The listing builds one solid part. Answer for the finished solid, in the listing's coordinates (mm). Face numbers are marked on the shaded views. A direction names the side the tool comes from. Round coordinates to 2 decimals unless told otherwise and drop trailing zeros. Order: outer loops, then holes, each group sorted by start corner. A loop starts at its lowest first (then second) coordinate and runs counter-clockwise, first axis right, second up. Notation, with made-up numbers: (33, 43) - (47, 43) arc R19 ccw to (47, 73) - close; hole circle Ø10 at (-27.75, -23). An arc over 180 degrees is marked (long way). One line per item, written item: value. Start each with the question number.
1. For a pull along X with two mould halves and no side action, classify the marked faces 1, 2 and 3 as released by +X, released by -X, zero draft, split by the parting line, or undercut.
2. Section A-A, the plane x = 0 is taken. Give the vertices of the cut face in (y, z), then the cut area to 3 significant figures.
3. A tool of negligible diameter and unlimited length cuts with its end or side. For the marked faces 4 and 5, from which of +Z, -Z, +X, -X, +Y, -Y can it reach the whole face along a straight path? Write none if from no direction.
4. Flat-ended cylindrical pins translate along their axes: P1, Ø5, axis at x = 1.5, y = 9.5, coming from the -Z side; P2, Ø2, axis at y = 11.5, z = 0.5, coming from the -X side; P3, Ø1.5, axis at x = 2.5, y = 6.5, coming from the -Z side. Find the tip coordinate at first contact, or state that the pin passes through.
5. Straight lines are drawn through the part: line 1 (Y direction, x = -1, z = 3.5); line 2 (Y direction, x = 1.5, z = 0.25); line 3 (X direction, y = 15.5, z = -2). For each, find the intervals that lie inside material, in ascending order.
6. Section B-B, the plane y = 7.5 is taken. Give the vertices of the cut face in (x, z).
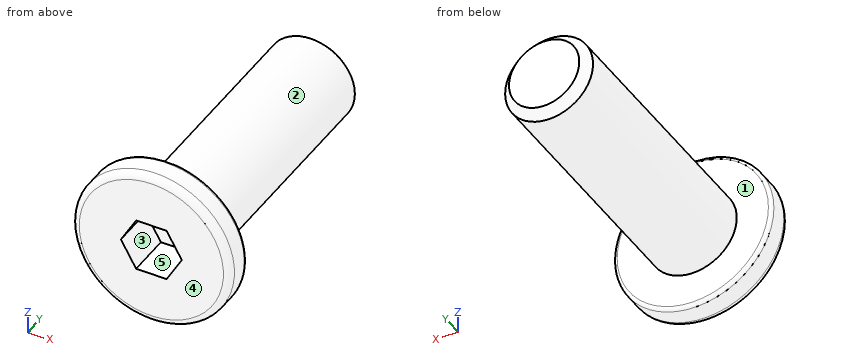
Autodesk Inventor part; units mm, degrees
ref_plane "YZ Plane" through (0, 0, 0) normal (1, 0, 0) x (0, 1, 0)
ref_plane "XZ Plane" through (0, 0, 0) normal (0, 1, 0) x (-1, 0, 0)
ref_plane "XY Plane" through (0, 0, 0) normal (0, 0, 1) x (1, 0, 0)
sketch "Boceto1" plane through (0, 0, 0) normal (0, 1, 0) x (-1, 0, 0)
  circle A0 centre (0, 0) radius 4.5
  dimension "d0" = 9
extrude "Extrusión1" add sketch "Boceto1" along normal blind 1.6
sketch "Boceto2" plane through (0, 1.6, 0) normal (0, 1, 0) x (1, 0, 0)
  circle A0 centre (0, 0) radius 2.5
  dimension "d3" = 5
extrude "Extrusión2" add sketch "Boceto2" along normal blind 15
fillet "Empalme1" radius 0.4 1 edges at (4.5, 0, 0)
fillet "Empalme2" radius 0.2 1 edges at (4.5, 1.6, 0)
sketch "Boceto3" plane through (0, 0, 0) normal (0, -1, 0) x (1, 0, 0)
  line L0 (-1.7321, 0) -> (-0.866, 1.5)
  line L1 (-0.866, 1.5) -> (0.866, 1.5)
  line L2 (0.866, 1.5) -> (1.7321, 0)
  line L3 (1.7321, 0) -> (0.866, -1.5)
  line L4 (0.866, -1.5) -> (-0.866, -1.5)
  line L5 (-0.866, -1.5) -> (-1.7321, 0)
  point P0 (0, 0)
  point P1 (0, 0)
  dimension "d8" = 3
extrude "Extrusión3" cut sketch "Boceto3" against normal blind 2.5
chamfer "Chaflán1" distance 0.5 angle 45 1 edges at (-2.5, 16.6, 0)
thread "Rosca2"
properties part number "Perno M5x15 cabeza plana_" material "Hierro, gris"
Answer list:
1. face 1: zero draft
1. face 2: split by the parting line
1. face 3: undercut
2. outline: (0, -4.1) arc R0.4 ccw to (0.4, -4.5) - (1.4, -4.5) arc R0.2 ccw to (1.6, -4.3) - (1.6, -2.5) - (16.1, -2.5) - (16.6, -2) - (16.6, 2) - (16.1, 2.5) - (1.6, 2.5) - (1.6, 4.3) arc R0.2 ccw to (1.4, 4.5) - (0.4, 4.5) arc R0.4 ccw to (0, 4.1) - (0, 1.5) - (2.5, 1.5) - (2.5, -1.5) - (0, -1.5) - close
2. area: 81.6 mm²
3. face 4: +Z, -Z, +X, -X, -Y
3. face 5: -Y
4. P1: stops at z = -2.5
4. P2: stops at x = -2.5
4. P3: stops at z = -1.79
5. line 1: y = 0 to 1.6
5. line 2: y = 2.5 to 16.6
5. line 3: x = -1.5 to 1.5
6. outline: circle Ø5 at (0, 0)
